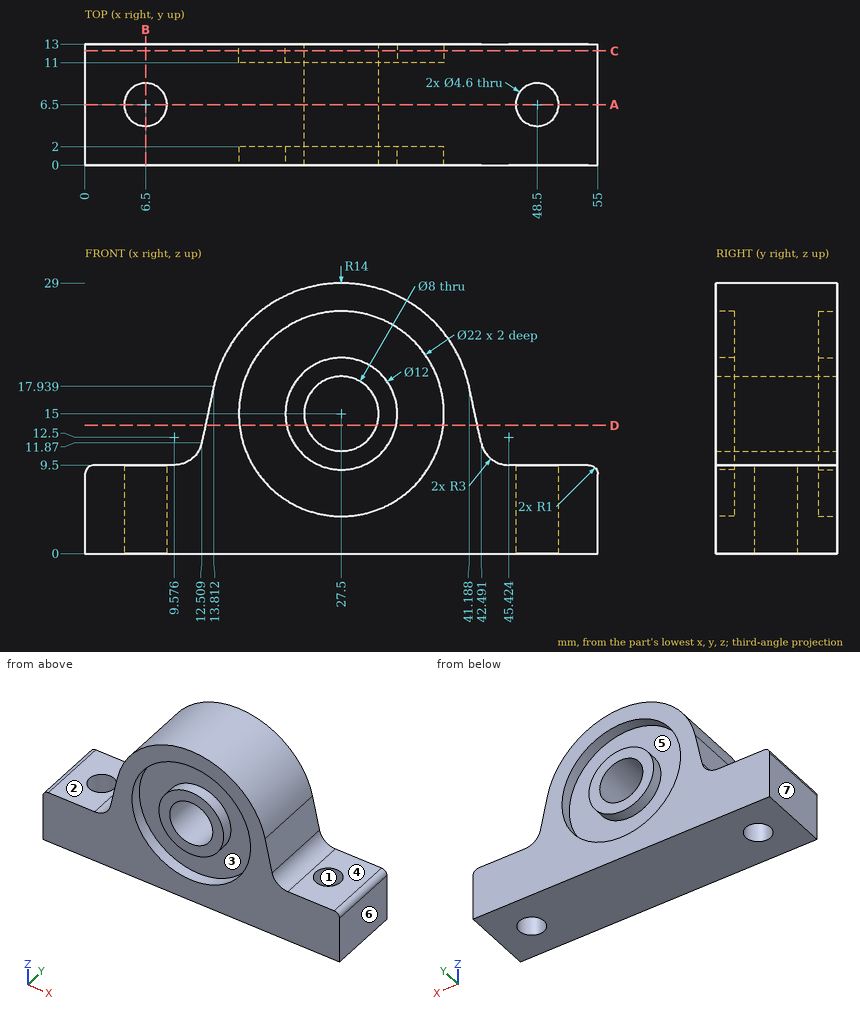
Print and shaded views of the part. All mm, measured from the part's lowest x, y and z. A direction names the side the tool comes from. Round coordinates to 2 decimals unless told otherwise and drop trailing zeros. Write each loop counter-clockwise with the first axis right and the second up, starting at its lowest first coordinate (ties: lowest second). Pieces come first, ordered by that corner, then holes. Notation, with made-up numbers: (53, 45) - (76, 45) arc R21 cw to (76, 57) - close; hole circle Ø6 at (31, -16). An arc over 180 degrees is marked (long way). Use CSV: the item, a comma, the result in double quotes. Start each with the question number.
Item 1: Drill centre lines: L1, parallel to Z at x = 27.5, y = 0.95; L2, parallel to Z at x = 27.5, y = 8.5; L3, parallel to X at y = 12.5, z = 10.25 (1 decimal). Where is each one in solid material? Low to high. Write a range as [from, to].
Item 2: Band-saw the part on B-B (x = 6.5). Write the cut outline in (y, z), and give its area (3 significant figures).
Item 3: Two-plate mould, pull along X, no slides. Class the marked faces 4, 5, 6 and 7: released by +X, released by -X, zero draft, split by the parting line, or undercut.
Item 4: Tool access for the marked faces 1, 2 and 3: list every direction of +Z, -Z, +X, -X, +Y, -Y with a clear straight run to the whole face (end or side of a thin tool).
Item 5: Pin check, flat tips, straight feed: P1, Ø3, axis at x = 22, y = 8.5, coming from the +Z side; P2, Ø5, axis at x = 27.5, z = 15, coming from the -Y side; P3, Ø4, axis at x = 40.5, y = 4, coming from the +Z side; P4, Ø4, axis at y = 4.5, z = 12, coming from the -X side (1 decimal). Stop position of each tip, or through.
Item 6: Band-saw the part on A-A (y = 6.5). Write the cut outline in (x, z), and give its area (3 significant figures).
Item 7: Band-saw the part on C-C (y = 12.25). Write the cut outline in (x, z).
Item 8: Band-saw the part on D-D (z = 13.75). Write the cut outline in (x, y).
Checked values:
1,L1,"z = [0, 4], [9, 11], [19, 21], [26, 29]"
1,L2,"z = [0, 11], [19, 29]"
1,L3,"x = [11.6, 17.6], [23.8, 31.2], [37.4, 43.4]"
2,outline,"(0, 0) - (4.2, 0) - (4.2, 9.5) - (0, 9.5) - close; (8.8, 0) - (13, 0) - (13, 9.5) - (8.8, 9.5) - close"
2,area,"79.8 mm²"
3,face 4,"zero draft"
3,face 5,"undercut"
3,face 6,"released by +X"
3,face 7,"released by -X"
4,face 1,"+Z, -Z"
4,face 2,"+Z, -X, +Y, -Y"
4,face 3,"-Y"
5,P1,"stops at z = 28.42"
5,P2,"passes through"
5,P3,"stops at z = 23.66"
5,P4,"stops at x = 11.2"
6,outline,"(0, 0) - (4.2, 0) - (4.2, 9.5) - (1, 9.5) arc R1 ccw to (0, 8.5) - close; (8.8, 0) - (46.2, 0) - (46.2, 9.5) - (45.42, 9.5) arc R3 cw to (42.49, 11.87) - (41.19, 17.94) arc R14 ccw to (13.81, 17.94) - (12.51, 11.87) arc R3 cw to (9.58, 9.5) - (8.8, 9.5) - close; (50.8, 0) - (55, 0) - (55, 8.5) arc R1 ccw to (54, 9.5) - (50.8, 9.5) - close; hole circle Ø8 at (27.5, 15)"
6,area,"859 mm²"
7,outline,"(0, 0) - (55, 0) - (55, 8.5) arc R1 ccw to (54, 9.5) - (45.42, 9.5) arc R3 cw to (42.49, 11.87) - (41.19, 17.94) arc R14 ccw to (13.81, 17.94) - (12.51, 11.87) arc R3 cw to (9.58, 9.5) - (1, 9.5) arc R1 ccw to (0, 8.5) - close; circle Ø12 at (27.5, 15); hole circle Ø22 at (27.5, 15); hole circle Ø8 at (27.5, 15)"
8,outline,"(12.91, 0) - (16.57, 0) - (16.57, 2) - (21.63, 2) - (21.63, 0) - (23.7, 0) - (23.7, 13) - (21.63, 13) - (21.63, 11) - (16.57, 11) - (16.57, 13) - (12.91, 13) - close; (31.3, 0) - (33.37, 0) - (33.37, 2) - (38.43, 2) - (38.43, 0) - (42.09, 0) - (42.09, 13) - (38.43, 13) - (38.43, 11) - (33.37, 11) - (33.37, 13) - (31.3, 13) - close"
